Autodesk Inventor part; units mm, degrees
ref_plane "Work Plane1" through (11.4, 0, 0) normal (1, 0, 0) x (0, 0, -1)
ref_plane "YZ Plane" through (0, 0, 0) normal (1, 0, 0) x (0, 1, 0)
ref_plane "XZ Plane" through (0, 0, 0) normal (0, 1, 0) x (-1, 0, 0)
sketch "Sketch1" plane through (0, 0, 0) normal (0, 0, 1) x (1, 0, 0)
  line L0 (0, 0) -> (22.8, 0)
  line L1 (22.8, 0) -> (22.8, 12.5)
  line L2 (22.8, 12.5) -> (0, 12.5)
  line L3 (0, 12.5) -> (0, 0)
  dimension "d0" = 22.8
  dimension "d1" = 12.5
extrude "Extrusion1" add sketch "Sketch1" along normal blind 22.1
sketch "Sketch2" plane through (22.8, 0, 0) normal (1, 0, 0) x (0, 0, -1)
  line L0 (0, 12.5) -> (-22.1, 12.5)
  line L1 (-22.1, 0) -> (-22.1, 12.5)
  line L2 (0, 0) -> (-22.1, 0)
  line L3 (-18, 12.5) -> (-15.6, 12.5)
  line L4 (-15.6, 12.5) -> (-15.6, 0)
  line L5 (-15.6, 0) -> (-18, 0)
  line L6 (-18, 0) -> (-18, 12.5)
  dimension "d4" = 2.4
  dimension "d5" = 4.1
extrude "Extrusion2" add sketch "Sketch2" along normal blind 4.8 contours L4 L2 L6 L0
sketch "Sketch3" plane through (22.8, 0, 18) normal (0, 0, 1) x (1, 0, 0)
  line L0 (0, 0) -> (0, 12.5)
  circle A0 centre (2.9, 6.25) radius 1
  point P0 (-22.8, 0)
  dimension "d8" = 2
  dimension "d9" = 2.9
extrude "Extrusion3" cut sketch "Sketch3" against normal up to surface (2.4 mm away)
sketch "Sketch4" plane through (27.6, 0, 0) normal (1, 0, 0) x (0, 0, -1)
  line L0 (-18, 12.5) -> (-18, 0)
  line L1 (-15.6, 0) -> (-15.6, 12.5)
  line L2 (-18, 6.85) -> (-15.6, 6.85)
  line L3 (-15.6, 6.85) -> (-15.6, 5.65)
  line L4 (-15.6, 5.65) -> (-18, 5.65)
  line L5 (-18, 5.65) -> (-18, 6.85)
  point P0 (0, 0)
  point P1 (-15.6, 6.25)
  point P2 (-15.6, 6.25)
  dimension "d12" = 1.2
extrude "Extrusion4" cut sketch "Sketch4" against normal blind 2
ref_plane "Work Plane1" through (11.4, 0, 0) normal (1, 0, 0) x (0, 0, -1)
mirror "Mirror1" about plane through (11.4, 0, 0) normal (1, 0, 0) of "Extrusion2", "Extrusion3", "Extrusion4"
sketch "Sketch5" plane through (0, 0, 22.1) normal (0, 0, 1) x (1, 0, 0)
  line L0 (0, 0) -> (22.8, 0)
  line L1 (22.8, 0) -> (22.8, 12.5)
  line L2 (0, 12.5) -> (0, 0)
  arc A0 (11.8625, 9) -> (11.8625, 3.5) centre (6.25, 6.25) ccw
  arc A1 (12.8, 3.5) -> (12.8, 9) centre (12.8, 6.25) ccw
  line L3 (12.8, 9) -> (11.8625, 9)
  line L4 (12.8, 3.5) -> (11.8625, 3.5)
  point P0 (0, 6.25)
  dimension "d16" = 5.5
  dimension "d17" = 10
extrude "Extrusion5" add sketch "Sketch5" along normal blind 4.1 contours A0 L3 A1 L4
sketch "Sketch6" plane through (0, 0, 26.2) normal (0, 0, 1) x (1, 0, 0)
  arc A0 (11.8625, 9) -> (11.8625, 3.5) centre (6.25, 6.25) ccw
  circle A1 centre (6.25, 6.25) radius 2.45
  point P0 (0, 0)
  dimension "d20" = 4.9
extrude "Extrusion6" add sketch "Sketch6" along normal blind 2.9
properties part number "Servo"
Verification items for the finished model (mm, model axes). A direction names the side the tool comes from. Give positions to 0.01 mm unless a question says otherwise; leave off trailing zeros. Loops run counter-clockwise (first coordinate to the right, second up) from the corner with the lowest first, then second, coordinate; pieces in that order, holes last.
1) Sectioned sample at D-D, the plane x = 22. Enter the section's corners in (y, z).
2) Set-up check for faces 1 (the flat face through (27, 6.85, 17)), 2 (the flat face through (0, 6, 20)), 3 (the cylindrical face through (15.55, 6.31, 24.12)): record each of +Z, -Z, +X, -X, +Y, -Y from which the full face is reachable in a straight line by a thin tool's end or side.
3) Draft check along Y on faces 4 (the flat face through (-4, 6.85, 17)), 5 (the flat face through (22.8, 6, 8)), 6 (the flat face through (12.3, 9, 24.1)). Enter one of: pulls with the +Y half, pulls with the -Y half, needs draft (parallel to the pull), parting line crosses it, or undercut.
4) Depth check by flat-ended pin: pin 1 Ø2 at (y, z) = (2, 22) entering from -X; pin 2 Ø1.9 at (x, y) = (2, 3) entering from +Z; pin 3 Ø4 at (y, z) = (5, 11.5) entering from +X. Enter the tip coordinate at first touch or a pass-through.
5) Thickness scan on line 1 along Y through (x, z) = (25.7, 16.2); line 2 along X through (y, z) = (6.25, 16.5); line 3 along Z through (x, y) = (13, 5.75). Record the ranges inside material, lowest first.
6) Sectioned sample at C-C, the plane z = 6.25. Enter the section's corners in (x, y), then the cut area to 3 significant figures.
7) Sectioned sample at A-A, the plane x = 25.7. Enter the section's corners in (y, z).
8) Sectioned sample at B-B, the plane y = 1. Enter the section's corners in (x, z).
Answers:
1. outline: (0, 0) - (12.5, 0) - (12.5, 22.1) - (0, 22.1) - close
2. face 1: +Z, -Z, +X
2. face 2: +Z, -X, +Y, -Y
2. face 3: +Z, +X
3. face 4: undercut
3. face 5: needs draft
3. face 6: pulls with the +Y half
4. pin 1: stops at x = 0
4. pin 2: stops at z = 26.2
4. pin 3: stops at x = 22.8
5. line 1: y = 0 to 5.25, 7.25 to 12.5
5. line 2: x = -1.9 to 24.7
5. line 3: z = 0 to 26.2
6. outline: (0, 0) - (22.8, 0) - (22.8, 12.5) - (0, 12.5) - close
6. area: 285 mm2
7. outline: (0, 15.6) - (5.25, 15.6) - (5.25, 18) - (0, 18) - close; (7.25, 15.6) - (12.5, 15.6) - (12.5, 18) - (7.25, 18) - close
8. outline: (-4.8, 15.6) - (0, 15.6) - (0, 0) - (22.8, 0) - (22.8, 15.6) - (27.6, 15.6) - (27.6, 18) - (22.8, 18) - (22.8, 22.1) - (9.64, 22.1) - (9.64, 26.2) - (2.86, 26.2) - (2.86, 22.1) - (0, 22.1) - (0, 18) - (-4.8, 18) - close
